Can you work these out from the model? Positions are in its coordinate system, mm. A direction names the side the tool comes from. Round coordinates to 2 decimals unless told otherwise and drop trailing zeros. Order: outer loops, then holes, each group sorted by start corner. A loop starts at its lowest first (then second) coordinate and runs counter-clockwise, first axis right, second up. Notation, with made-up numbers: M -30.75,13 L -22.75,13 A21 cw -22.75,17 Z; hole C -35,78 d5. An arc over 180 degrees is marked long. Answer as CSV lines item,"result". Start each with the question number.
from build123d import *

# Parameters (mm, degrees)
SKETCH1_W                               = 140
SKETCH1_H                               = 20
SKETCH1_W_2                             = 5
SKETCH1_H_2                             = 12
BOSS_EXTRUDE1_DEPTH                     = 2.5
SKETCH2_R                               = 5
CUT_EXTRUDE1_DEPTH                      = 5
M3_TAPPED_HOLE2_D                       = 2.5
M3_TAPPED_HOLE2_CSINK_D                 = 3.05
M3_TAPPED_HOLE2_CSINK_ANGLE             = 90
F_5_0MM_DOWEL_HOLE1_D                   = 5
CBORE_FOR_M5_HEX_HEAD_BOLT2_D           = 3
CBORE_FOR_M5_HEX_HEAD_BOLT2_CBORE_D     = 4
CBORE_FOR_M5_HEX_HEAD_BOLT2_CBORE_DEPTH = 3
CUT_EXTRUDE2_DEPTH                      = 10


with BuildPart() as part:
    # Sketch1 → Boss-Extrude1 (new, symmetric)
    with BuildSketch(Plane(origin=(0, 0, 0), x_dir=(1, 0, 0), z_dir=(0, 1, 0))):
        Rectangle(SKETCH1_W, SKETCH1_H)
        with Locations((72.5, 0)):
            Rectangle(SKETCH1_W_2, SKETCH1_H_2)
    extrude(amount=BOSS_EXTRUDE1_DEPTH, both=True)

    # Sketch2 → Cut-Extrude1 (cut)
    with BuildSketch(Plane.XZ.offset(2.5)):
        with Locations(Location((48, 0, 0), (0, 0, 270))):
            Circle(SKETCH2_R)
    extrude(amount=-CUT_EXTRUDE1_DEPTH, mode=Mode.SUBTRACT)

    # M3 Tapped Hole2 (through all)
    with Locations(Plane(origin=(0, -2.5, 0), x_dir=(-1, 0, 0), z_dir=(0, -1, 0))):
        with Locations((-56, 6), (-40, 6), (-40, -6), (-56, -6)):
            CounterSinkHole(M3_TAPPED_HOLE2_D / 2, M3_TAPPED_HOLE2_CSINK_D / 2, counter_sink_angle=M3_TAPPED_HOLE2_CSINK_ANGLE)

    # Ø5.0mm Dowel Hole1 (through all)
    with Locations(Plane(origin=(0, -2.5, 0), x_dir=(-1, 0, 0), z_dir=(0, -1, 0))):
        with Locations((4, 0)):
            Hole(F_5_0MM_DOWEL_HOLE1_D / 2)

    # CBORE for M5 Hex Head Bolt2 (through all)
    with Locations(Plane(origin=(-16.649110641, 2.5, 3), x_dir=(0, 0, 1), z_dir=(0, 1, 0))):
        with Locations((0, 0), (-6, 0)):
            CounterBoreHole(CBORE_FOR_M5_HEX_HEAD_BOLT2_D / 2, CBORE_FOR_M5_HEX_HEAD_BOLT2_CBORE_D / 2, CBORE_FOR_M5_HEX_HEAD_BOLT2_CBORE_DEPTH)

    # Sketch29 → Cut-Extrude2 (cut)
    with BuildSketch(Plane(origin=(0, 2.5, 0), x_dir=(1, 0, 0), z_dir=(0, 1, 0))):
        with BuildLine():
            ThreePointArc((-28, -10), (-30, 0), (-28, 10))
            Line((-28, 10), (-70, 10))
            Line((-70, 10), (-70, -10))
            Line((-70, -10), (-28, -10))
        make_face()
    extrude(amount=-CUT_EXTRUDE2_DEPTH, mode=Mode.SUBTRACT)


solid = part.part
(1) If I drill on line 1 along X through (y, z) = (-0.9, -0.25); line 2 along Z through (x, y) = (56, 0.2); line 3 along X through (y, z) = (0.8, -3), over which ranges is the centre line in solid material (lowest first)?
(2) I want a section at B-B on z = 0. Write out the boundary of the cut face in (x, y), and give its area (3 significant figures).
(3) I want a section at C-C on x = -4. Write out the boundary of the cut face in (y, z), and give its area (3 significant figures).
(4) For faces 1 (the cylindrical face through (-1.615, 0.035, -0.751)), 2 (the cylindrical face through (-17.866, 1.021, 1.413)), 3 (the flat face through (72, 0, 6)), which set-ups out of +Z, -Z, +X, -X, +Y, -Y let a thin tool reach every point of the face, with its end or its side?
(5) I'm going to push a flat-ended pin straight in: P1, Ø1.5, axis at x = 73, y = 0, coming from the -Z side. Where does the tip first touch, or does it pass through?
(6) I want a section at D-D on y = 0.75. Count the separate pieces of the cut face and the enclosed holes in it, and give its area (3 significant figures).
(7) If we mould it in two halves opening along X, with no side actions, what happens to faces 4 (the flat face through (72, 0, -6)), 5 (the cylindrical face through (57.19, 0.17, 5.62)), 6 (the flat face through (70, 0, -8))? For each: +X half, -X half, draft (parallel to the pull), parting line (faces both ways), or undercut.
(8) I want a section at A-A on x = 56. Write out the boundary of the cut face in (y, z) (3 decimals), and give its area (3 significant figures).
From the geometry:
1,line 1,"-30 to -6.49, -1.51 to 43.01, 52.99 to 75"
1,line 2,"-10 to -7.25, -4.75 to 4.75, 7.25 to 10"
1,line 3,"-29.83 to -18.65, -14.65 to 44, 52 to 75"
2,outline,"M -30,-2.5 L -6.5,-2.5 L -6.5,2.5 L -30,2.5 Z; M -1.5,-2.5 L 43,-2.5 L 43,2.5 L -1.5,2.5 Z; M 53,-2.5 L 75,-2.5 L 75,2.5 L 53,2.5 Z"
2,area,"450 mm²"
3,outline,"M -2.5,-10 L 2.5,-10 L 2.5,-2.5 L -2.5,-2.5 Z; M -2.5,2.5 L 2.5,2.5 L 2.5,10 L -2.5,10 Z"
3,area,"75.0 mm²"
4,face 1,"+Y, -Y"
4,face 2,"+Y"
4,face 3,"+Z, +X, +Y, -Y"
5,P1,"z = -6"
6,separate pieces,"1"
6,enclosed holes,"8"
6,area,"1,900 mm²"
7,face 4,"draft"
7,face 5,"undercut"
7,face 6,"+X half"
8,outline,"M -2.5,-10 L 2.5,-10 L 2.5,-7.25 L -2.225,-7.25 L -2.5,-7.525 Z; M -2.5,-4.475 L -2.225,-4.75 L 2.5,-4.75 L 2.5,4.75 L -2.225,4.75 L -2.5,4.475 Z; M -2.5,7.525 L -2.225,7.25 L 2.5,7.25 L 2.5,10 L -2.5,10 Z"
8,area,"74.8 mm²"
